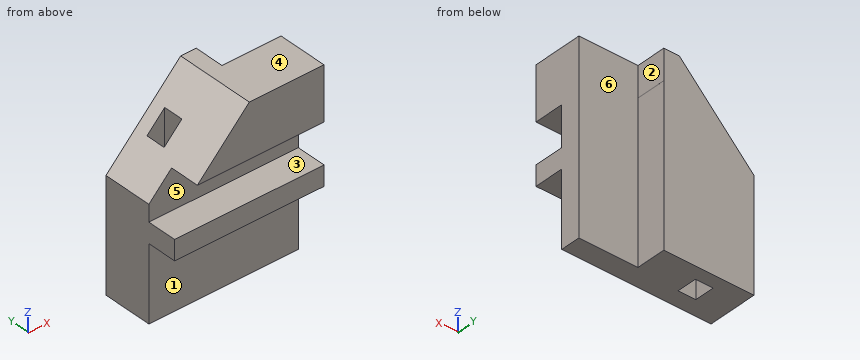
Solid Edge part; units mm, degrees
sketch "Sketch1" plane through (0, 0, 0) normal (0, -1, 0) x (1, 0, 0)
  line L0 (0, 0) -> (0, 67)
  line L1 (45, 113) -> (0, 67)
  line L2 (90, 113) -> (45, 113)
  line L3 (90, 0) -> (90, 113)
  line L4 (0, 0) -> (90, 0)
extrude "Protrusion1" add sketch "Sketch1" against normal blind 48
sketch "Sketch2" plane through (0, 24, 33.5) normal (-1, 0, 0) x (0, -1, 0)
  line L0 (6, 47.5) -> (31.2141, 47.5)
  line L1 (31.2141, 23.5) -> (31.2141, 47.5)
  line L2 (6, 23.5) -> (31.2141, 23.5)
  line L3 (6, 23.5) -> (6, 47.5)
extrude "ExtrudedCutout_5" cut sketch "Sketch2" against normal blind 119.7329
sketch "Sketch3" plane through (0, 24, 33.5) normal (-1, 0, 0) x (0, -1, 0)
  line L0 (24, 11.5) -> (6, 11.5)
  line L1 (6, 11.5) -> (6, -33.5)
  line L2 (6, -33.5) -> (6, -39.0842)
  line L3 (6, -39.0842) -> (32.5581, -39.0842)
  line L4 (32.5581, 11.5) -> (32.5581, -39.0842)
  line L5 (24, 11.5) -> (32.5581, 11.5)
extrude "ExtrudedCutout_7" cut sketch "Sketch3" against normal blind 121.1095
sketch "Sketch4" plane through (45, 24, 90) normal (-0.4551, 0, 0.8904) x (0, -1, 0)
  line L0 (-6, 50.5371) -> (-6, 10.5371)
  line L1 (-6, 10.5371) -> (-33.3902, 10.5371)
  line L2 (-33.3902, 10.5371) -> (-33.3902, 50.5371)
  line L3 (-33.3902, 50.5371) -> (-6, 50.5371)
extrude "ExtrudedCutout_8" cut sketch "Sketch4" against normal blind 192.3862
sketch "Sketch5" plane through (45, 33, 0) normal (0, 0, -1) x (0, -1, 0)
  line L0 (-7, 27.1913) -> (5, 27.1913)
  line L1 (5, 27.1913) -> (5, 16.5061)
  line L2 (5, 16.5061) -> (-7, 16.5061)
  line L3 (-7, 16.5061) -> (-7, 27.1913)
extrude "ExtrudedCutout_9" cut sketch "Sketch5" against normal blind 129.7045
sketch "Sketch6" plane through (67.5, 24, 113) normal (0, 0, 1) x (0, -1, 0)
  line L0 (-6, 22.5) -> (-6, -13.1174)
  line L1 (-6, -13.1174) -> (-33.3902, -13.1174)
  line L2 (-33.3902, -13.1174) -> (-33.3902, 22.5)
  line L3 (-33.3902, 22.5) -> (-6, 22.5)
extrude "ExtrudedCutout_10" cut sketch "Sketch6" against normal blind 144.9371
CAD build for the part. Positions are in the model's coordinates, mm. Face numbers are marked on the shaded views. A direction names the side the tool comes from. Round coordinates to 2 decimals unless told otherwise and drop trailing zeros. Order: outer loops, then holes, each group sorted by start corner. A loop starts at its lowest first (then second) coordinate and runs counter-clockwise, first axis right, second up. Notation, with made-up numbers: (4, -18.75) - (22, -18.75) arc R8 ccw to (22, -14.75) - close; hole circle Ø6 at (52, 83.25). An arc over 180 degrees is marked (long way). Answer as CSV lines item,"result". Start each with the question number.
1. Pull direction Z, two halves, no side cores. Call the marked faces 4, 5 and 6: +Z half, -Z half, draft (parallel to the pull), parting line (faces both ways), or undercut.
2. Saw through at C-C, the plane x = 25. Write the cut outline in (y, z).
3. Pin check, flat tips, straight feed: pin 1 (5 mm diameter, centred on x = 26.5, y = 41, fed in from +Z); pin 2 (5 mm diameter, centred on y = 40, z = 48.5, fed in from +X); pin 3 (5.5 mm diameter, centred on x = 42, y = 8, fed in from +Z). Stop position of each tip, or through.
4. Drill centre lines: L1, parallel to Z at x = 80.5, y = 5.5; L2, parallel to X at y = 31, z = 38.5; L3, parallel to Y at x = 48, z = 37. Where is each one in solid material? Low to high. Write a range as [from, to].
5. Saw through at D-D, the plane x = 51.5. Write the cut outline in (y, z).
6. Tool access for the marked faces 1, 2 and 3: list every direction of +Z, -Z, +X, -X, +Y, -Y with a clear straight run to the whole face (end or side of a thin tool).
7. Saw through at A-A, the plane z = 35.5. Write the cut outline in (x, y).
Model answer:
1,face 4,"+Z half"
1,face 5,"undercut"
1,face 6,"draft"
2,outline,"(0, 45) - (18, 45) - (18, 0) - (28, 0) - (28, 92.56) - (0, 92.56) - (0, 81) - (18, 81) - (18, 57) - (0, 57) - close; (40, 0) - (48, 0) - (48, 92.56) - (40, 92.56) - close"
3,pin 1,"stops at z = 96.64"
3,pin 2,"stops at x = 54.38"
3,pin 3,"stops at z = 112.74"
4,L1,"z = [45, 57], [81, 113]"
4,L2,"x = [0, 17.81], [28.49, 54.38]"
4,L3,"y = [18, 48]"
5,outline,"(0, 45) - (18, 45) - (18, 0) - (48, 0) - (48, 113) - (0, 113) - (0, 81) - (18, 81) - (18, 57) - (0, 57) - close"
6,face 1,"-Z, +X, -X, -Y"
6,face 2,"+Z, -Z, +X, +Y"
6,face 3,"+X, -X, -Y"
7,outline,"(0, 18) - (90, 18) - (90, 30) - (54.38, 30) - (54.38, 48) - (0, 48) - close; hole (17.81, 28) - (28.49, 28) - (28.49, 40) - (17.81, 40) - close"
